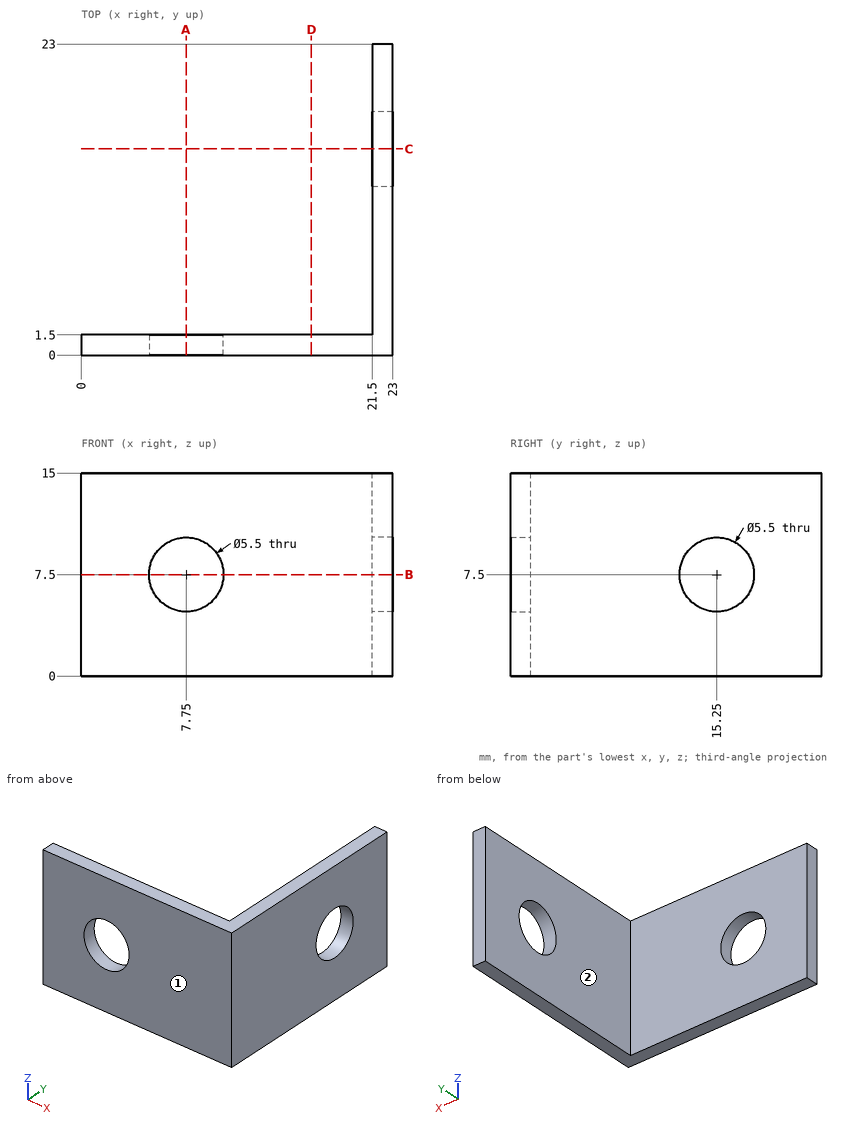
Could you check a few things on this drawing? It's one solid part, dimensions in mm from its lowest x, y, z. A direction names the side the tool comes from. Give positions to 0.01 mm unless a question says otherwise; leave off trailing zeros. Write each loop counter-clockwise with the first axis right and the second up, starting at its lowest first coordinate (ties: lowest second). Pieces come first, ordered by that corner, then holes. Notation, with made-up numbers: (73, -37) - (132, -37) arc R18 ccw to (132, -23) - close; hole circle Ø5 at (6, -4). An arc over 180 degrees is marked (long way). Use CSV: the item, a comma, the result in double quotes. Start each with the question number.
Item 1: I want a section at A-A, the plane x = 7.75. Please give me the cut outline in (y, z).
Item 2: I want a section at D-D, the plane x = 17. Please give me the cut outline in (y, z), then the cut area to 3 significant figures.
Item 3: For the marked faces 1 and 2, which set-ups out of +Z, -Z, +X, -X, +Y, -Y let a thin tool reach every point of the face, with its end or its side?
Item 4: I'm going to push flat-ended pins straight in: pin 1 (2 mm diameter, centred on x = 6, z = 8, fed in from +Y); pin 2 (4.5 mm diameter, centred on y = 14, z = 6.5, fed in from -X). Where does each tip first touch, or does it pass through?
Item 5: I want a section at B-B, the plane z = 7.5. Please give me the cut outline in (x, y).
Item 6: If I drill on line 1 along Z through (x, y) = (7.75, 0.3); line 2 along Y through (x, z) = (5.75, 2.25); line 3 along X through (y, z) = (10.25, 11.75), over which ranges is the centre line in solid material (lowest first)?
Item 7: I want a section at C-C, the plane y = 15.25. Please give me the cut outline in (x, z), then the cut area to 4 significant figures.
Findings:
1,outline,"(0, 0) - (1.5, 0) - (1.5, 4.75) - (0, 4.75) - close; (0, 10.25) - (1.5, 10.25) - (1.5, 15) - (0, 15) - close"
2,outline,"(0, 0) - (1.5, 0) - (1.5, 15) - (0, 15) - close"
2,area,"22.5 mm2"
3,face 1,"+Z, -Z, +X, -X, -Y"
3,face 2,"+Z, -Z, -X, +Y"
4,pin 1,"stops at y = 1.5"
4,pin 2,"stops at x = 21.5"
5,outline,"(0, 0) - (5, 0) - (5, 1.5) - (0, 1.5) - close; (10.5, 0) - (23, 0) - (23, 12.5) - (21.5, 12.5) - (21.5, 1.5) - (10.5, 1.5) - close; (21.5, 18) - (23, 18) - (23, 23) - (21.5, 23) - close"
6,line 1,"z = 0 to 4.75, 10.25 to 15"
6,line 2,"y = 0 to 1.5"
6,line 3,"x = 21.5 to 23"
7,outline,"(21.5, 0) - (23, 0) - (23, 4.75) - (21.5, 4.75) - close; (21.5, 10.25) - (23, 10.25) - (23, 15) - (21.5, 15) - close"
7,area,"14.25 mm2"
